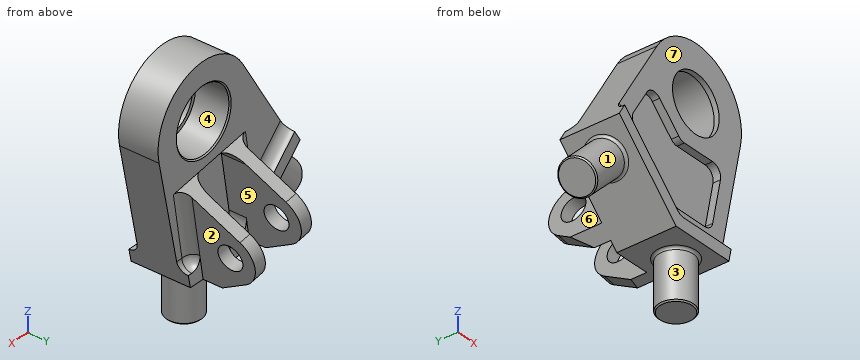
from build123d import *

# Parameters (mm, degrees)
SZKIC1_R                        = 13
SZKIC1_R_2                      = 11.5
DODANIE_WYCI_GNI_CIE1_DEPTH     = 8
SZKIC2_R                        = 5.0000000000000036
DODANIE_WYCI_GNI_CIE2_DEPTH     = 14
DODANIE_WYCI_GNI_CIE3_DEPTH     = 12
WYTNIJ_WYCI_GNI_CIE1_DEPTH      = 81.41142519817177
WYTNIJ_WYCI_GNI_CIE1_DEPTH_BACK = 6
SZKIC1_3_R                      = 13
SZKIC1_3_R_2                    = 11.5
WYTNIJ_WYCI_GNI_CIE2_DEPTH      = 78.26575763170368
WYTNIJ_WYCI_GNI_CIE2_DEPTH_BACK = 3
WYTNIJ_WYCI_GNI_CIE3_START      = 4
WYTNIJ_WYCI_GNI_CIE3_DEPTH      = 74.265757666648
WYTNIJ_WYCI_GNI_CIE4_DEPTH      = 78.26575763170368
SZKIC4_R                        = 7
DODANIE_WYCI_GNI_CIE4_DEPTH     = 20
SZKIC5_R                        = 7
DODANIE_WYCI_GNI_CIE5_DEPTH     = 20
WYTNIJ_WYCI_GNI_CIE5_DEPTH      = 3
ZAOKR_GLENIE1_R                 = 4
ZAOKR_GLENIE2_R                 = 4
ZAOKR_GLENIE3_R                 = 1
SFAZOWANIE1_SIZE                = 0.5


with BuildPart() as part:
    # Szkic1 → Dodanie-wyciągnięcie1 (new, symmetric)
    # profile 1 of 2: a face of its own
    with BuildSketch(Plane(origin=(0, 0, 0), x_dir=(1, 0, 0), z_dir=(0, 1, 0))):
        with BuildLine():
            Line((-39.9157635445463, 22.238094014882595), (-19.20964530804123, -11.714927534528307))
            ThreePointArc((-19.20964530804123, -11.714927534528307), (8.303589569253562, -20.911728772757726), (22.01344157137967, 4.653857559428904))
            Line((22.01344157137967, 4.653857559428904), (12.499999999999995, 49.6538575594289))
            Line((12.499999999999995, 49.6538575594289), (-12.499999999999995, 49.6538575594289))
            Line((-12.499999999999995, 49.6538575594289), (-39.9157635445463, 22.238094014882595))
        make_face()
        Circle(SZKIC1_R, mode=Mode.SUBTRACT)
    # profile 2 of 2: a face of its own
    with BuildSketch(Plane(origin=(0, 0, 0), x_dir=(1, 0, 0), z_dir=(0, 1, 0))):
        Circle(SZKIC1_R)
        with Locations(Location((0, 0, 0), (0, 0, 270))):
            Circle(SZKIC1_R_2, mode=Mode.SUBTRACT)
    extrude(amount=DODANIE_WYCI_GNI_CIE1_DEPTH, both=True)

    # Szkic2 → Dodanie-wyciągnięcie2 (add, symmetric)
    with BuildSketch(Plane(origin=(0, 0, 0), x_dir=(-0.16204203158770583, 0, -0.9867838567786408), z_dir=(0.9867838567786409, 0, -0.16204203158770586))):
        with BuildLine():
            Line((17.185981887192586, 8), (29.887687809364394, 30.00000000000001))
            ThreePointArc((29.887687809364394, 30.00000000000001), (38.54794184720877, 35), (47.20819588505315, 30.000000000000014))
            Line((47.20819588505315, 30.000000000000014), (57.02315046127683, 13.000000000000002))
            Line((57.02315046127683, 13.000000000000002), (57.02315046127683, 8))
            Line((57.02315046127683, 8), (17.185981887192586, 8))
        make_face()
        with Locations((38.54794184720877, 25)):
            Circle(SZKIC2_R, mode=Mode.SUBTRACT)
    extrude(amount=DODANIE_WYCI_GNI_CIE2_DEPTH, both=True)

    # Szkic1<5> → Dodanie-wyciągnięcie3 (add, symmetric)
    with BuildSketch(Plane(origin=(0, 0, 0), x_dir=(1, 0, 0), z_dir=(0, 1, 0))):
        Polygon((-12.499999999999995, 49.6538575594289), (12.499999999999995, 49.6538575594289), (11.442950936513364, 54.6538575594289), (-14.571067811865477, 54.6538575594289), (-42.59444393988905, 26.630481431405318), (-39.9157635445463, 22.238094014882595), align=None)
    extrude(amount=DODANIE_WYCI_GNI_CIE3_DEPTH, both=True)

    # Szkic1<3> → Wytnij-wyciągnięcie1 (cut, two sides: drawn at the far end of the back side and taken through both)
    with BuildSketch(Plane(origin=(0, 0, 0), x_dir=(1, 0, 0), z_dir=(0, 1, 0)).offset(-WYTNIJ_WYCI_GNI_CIE1_DEPTH_BACK)):
        with Locations(Location((0, 0, 0), (0, 0, 270))):
            Circle(SZKIC1_3_R)
        with Locations(Location((0, 0, 0), (0, 0, 270))):
            Circle(SZKIC1_3_R_2, mode=Mode.SUBTRACT)
    extrude(amount=WYTNIJ_WYCI_GNI_CIE1_DEPTH + WYTNIJ_WYCI_GNI_CIE1_DEPTH_BACK, mode=Mode.SUBTRACT)

    # Szkic3 → Wytnij-wyciągnięcie2 (cut, two sides: drawn at the far end of the back side and taken through both)
    with BuildSketch(Plane(origin=(0, 8, 0), x_dir=(1, 0, 0), z_dir=(0, 1, 0)).offset(-WYTNIJ_WYCI_GNI_CIE2_DEPTH_BACK)):
        with BuildLine():
            Line((-16.080898850750692, 42.386356929210905), (-11.665906130837973, 15.500471204882405))
            Line((-11.665906130837973, 15.500471204882405), (6.096203291177561, 18.417227773461114))
            Line((6.096203291177559, 18.417227773461114), (0.9667649489300167, 49.6538575594289))
            Line((0.9667649489300163, 49.6538575594289), (-9.9094763840183, 49.6538575594289))
            ThreePointArc((-9.9094763840183, 49.6538575594289), (-14.676630164659013, 47.44795607994614), (-16.080898850750696, 42.386356929210905))
        make_face()
    extrude(amount=WYTNIJ_WYCI_GNI_CIE2_DEPTH + WYTNIJ_WYCI_GNI_CIE2_DEPTH_BACK, mode=Mode.SUBTRACT)

    # Szkic3<3> → Wytnij-wyciągnięcie3 (cut, through all)
    with BuildSketch(Plane(origin=(0, 8, 0), x_dir=(1, 0, 0), z_dir=(0, 1, 0)).offset(WYTNIJ_WYCI_GNI_CIE3_START)):
        with BuildLine():
            ThreePointArc((-16.080898850750696, 42.386356929210905), (-14.676630164659013, 47.44795607994614), (-9.9094763840183, 49.6538575594289))
            Line((-9.9094763840183, 49.6538575594289), (0.9667649489300167, 49.6538575594289))
            Line((0.9667649489300163, 49.6538575594289), (0.14570352562758648, 54.6538575594289))
            Line((0.14570352562758646, 54.6538575594289), (-14.571067811865477, 54.65385755942889))
            Line((-14.571067811865477, 54.65385755942889), (-17.59826945789091, 51.626655913403454))
            Line((-17.59826945789091, 51.626655913403454), (-16.080898850750696, 42.386356929210905))
        make_face()
    extrude(amount=WYTNIJ_WYCI_GNI_CIE3_DEPTH, mode=Mode.SUBTRACT)

    # Szkic3<4> → Wytnij-wyciągnięcie4 (cut, through all)
    with BuildSketch(Plane(origin=(0, 8, 0), x_dir=(1, 0, 0), z_dir=(0, 1, 0))):
        Polygon((-9.240147148276744, 56.26952433784747), (-8.97483481534258, 54.65385755942888), (0.14570352562758693, 54.6538575594289), (5.212669270611022, 54.6538575594289), (4.5748268466242505, 58.53811278007535), align=None)
        Polygon((-14.571067811865477, 54.65385755942889), (-8.974834815342582, 54.65385755942889), (-9.240147148276744, 56.26952433784747), (-23.055121143177697, 54.00093589561959), (-21.95053906691765, 47.274386304376705), (-17.59826945789091, 51.626655913403454), align=None)
    extrude(amount=WYTNIJ_WYCI_GNI_CIE4_DEPTH, mode=Mode.SUBTRACT)

    # Szkic4 → Dodanie-wyciągnięcie4 (add)
    with BuildSketch(Plane(origin=(0, 0, -54.6538575594289), x_dir=(-1, 0, 0), z_dir=(0, 0, -1))):
        Circle(SZKIC4_R)
    extrude(amount=DODANIE_WYCI_GNI_CIE4_DEPTH)

    # Szkic5 → Dodanie-wyciągnięcie5 (add)
    with BuildSketch(Plane(origin=(-34.6124626856472, 0, -34.61246268564717), x_dir=(-0.7071067811865475, 0, 0.7071067811865477), z_dir=(-0.7071067811865477, 0, -0.7071067811865475))):
        Circle(SZKIC5_R)
    extrude(amount=DODANIE_WYCI_GNI_CIE5_DEPTH)

    # Szkic6 → Wytnij-wyciągnięcie5 (cut)
    with BuildSketch(Plane.XZ.offset(8)):
        Polygon((7.635842149160336, -43.65385755942889), (13.165024277111744, -17.499999999999996), (-7.248737341529154, -17.5), (-21.380397649888803, -3.3683396916403576), (-32.335886609702584, -21.332689575487763), (-10.01471862576144, -43.65385755942889), align=None)
    extrude(amount=-WYTNIJ_WYCI_GNI_CIE5_DEPTH, mode=Mode.SUBTRACT)

    # Zaokrąglenie1
    zaokr_glenie1_edges = [part.edges().sort_by_distance(p)[0] for p in [
        (7.635842149160336, -6.5, -43.65385755942889),
        (-10.01471862576144, -6.5, -43.65385755942889),
        (-32.335886609702584, -6.5, -21.332689575487763),
        (-21.380397649888803, -6.5, -3.3683396916403576),
        (-7.248737341529154, -6.5, -17.5),
        (13.165024277111744, -6.5, -17.499999999999996),
        (-12.499999999999995, -10, -49.6538575594289),
        (6.033730693913451, 10, -49.6538575594289),
        (-20.953164090141588, 10, -41.20069346928731),
        (6.09620329117756, 6.5, -18.417227773461114),
        (0.9667649489300165, 8.5, -49.6538575594289),
        (-11.665906130837973, 6.5, -15.500471204882405),
    ]]
    fillet(zaokr_glenie1_edges, radius=ZAOKR_GLENIE1_R)

    # Zaokrąglenie2
    zaokr_glenie2_edges = [part.edges().sort_by_distance(p)[0] for p in [
        (-18.144884891779377, 8, -24.099176343644537),
        (-22.41182088800963, 8, -36.667644697134236),
        (-33.19063523261732, 8, -28.96322232681158),
        (11.622076214271065, 8, -49.6538575594289),
        (8.91356978824917, 8, -32.11656368223886),
        (7.695163046353066, 8, -48.2430009983481),
        (-26.793668209900048, -8, -35.360189349528845),
        (-12.373879479967972, -8, -49.34937568947405),
        (0.8284271247461916, -8, -49.6538575594289),
    ]]
    fillet(zaokr_glenie2_edges, radius=ZAOKR_GLENIE2_R - 0.0001)  # a hair under: the kernel refuses the full size

    # Zaokrąglenie3
    zaokr_glenie3_edges = [part.edges().sort_by_distance(p)[0] for p in [
        (7, 8.6e-16, -54.6538575594289),
        (-29.66271521734136, 8.6e-16, -39.56221015395302),
    ]]
    fillet(zaokr_glenie3_edges, radius=ZAOKR_GLENIE3_R)

    # Sfazowanie1
    sfazowanie1_edges = [part.edges().sort_by_distance(p)[0] for p in [
        (7, 8.6e-16, -74.6538575594289),
        (-43.804850841072316, 8.6e-16, -53.70434577768397),
        (6.57e-15, 8, -13),
    ]]
    chamfer(sfazowanie1_edges, length=SFAZOWANIE1_SIZE)


solid = part.part
The listing builds one solid part. Answer for the finished solid, in the listing's coordinates (mm). Face numbers are marked on the shaded views. A direction names the side the tool comes from. Round coordinates to 2 decimals unless told otherwise and drop trailing zeros. Write each loop counter-clockwise with the first axis right and the second up, starting at its lowest first coordinate (ties: lowest second). Pieces come first, ordered by that corner, then holes. Notation, with made-up numbers: (-29, 5.5) - (-16, 5.5) arc R33 cw to (-16, 42.5) - close; hole circle Ø11 at (14.25, 31.5). An arc over 180 degrees is marked (long way). Use one line per item in the form item = value. Start each with the question number.
Item 1: A cutting plane is placed at C-C (z = -67). Write down the section's boundary in (x, y), plus the area to 3 significant figures.
Item 2: Determine the mould class of the marked faces 1, 2, 3 and 4 for opening direction Z: +Z half, -Z half, draft (parallel to the pull), parting line (faces both ways), or undercut.
Item 3: Find the intervals of material crossed by line 1 (Z direction, x = 0, y = 4); line 2 (Z direction, x = 2, y = -5.5); line 3 (Y direction, x = -8.5, z = -15), in increasing order. Write a range as [from, to].
Item 4: A tool of negligible diameter and unlimited length cuts with its end or side. For the marked faces 5, 6 and 7, from which of +Z, -Z, +X, -X, +Y, -Y can it reach the whole face along a straight path? Write none if from no direction.
Item 5: A cutting plane is placed at B-B (z = 0). Write down the section's boundary in (x, y), plus the area to 3 significant figures.
Item 6: Flat-ended cylindrical pins translate along their axes: pin 1 Ø21 at (x, z) = (6, -4) entering from +Y; pin 2 Ø18 at (x, z) = (-10, -27.5) entering from +Y; pin 3 Ø10 at (x, z) = (-21, -32) entering from -Y. Find the tip coordinate at first contact, or state that the pin passes through.
Item 7: A cutting plane is placed at A-A (y = 0). Write down the section's boundary in (x, z).
The answers:
q1.outline = circle Ø14 at (0, 0)
q1.area = 154 mm^2
q2.face_1 = undercut
q2.face_2 = -Z half
q2.face_3 = draft
q2.face_4 = undercut
q3.line_1 = [-74.65, -13], [13, 22.5]
q3.line_2 = [-74.65, -43.65], [-17.5, -12.85], [12.85, 22.41]
q3.line_3 = [-8, 8]
q4.face_5 = +Y
q4.face_6 = +Z, -X, +Y
q4.face_7 = +Z, +X, -Y
q5.outline = (-26.35, -8) - (-11.5, -8) - (-11.5, -6) - (-13, -6) - (-13, 7.5) - (-13.5, 8) - (-26.35, 8) - close; (11.5, -8) - (22.5, -8) - (22.5, 8) - (13.5, 8) - (13, 7.5) - (13, -6) - (11.5, -6) - close
q5.area = 371 mm^2
q6.pin_1 = 8
q6.pin_2 = 34.88
q6.pin_3 = -8.9
q7.outline = (-53.35, -44.16) - (-44.16, -53.35) - (-43.45, -53.35) - (-30.37, -40.27) arc R1 cw to (-28.96, -40.27) - (-14.57, -54.65) - (-8, -54.65) arc R1 cw to (-7, -55.65) - (-7, -74.15) - (-6.5, -74.65) - (6.5, -74.65) - (7, -74.15) - (7, -55.65) arc R1 cw to (8, -54.65) - (11.44, -54.65) - (22.01, -4.65) arc R22.5 ccw to (-19.21, 11.71) - (-42.59, -26.63) - (-40.27, -28.96) arc R1 cw to (-40.27, -30.37) - (-53.35, -43.45) - close; hole circle Ø26 at (0, 0)
